```python
from build123d import *

# Parameters (mm, degrees)
F0_R     = 136.525
F0_R_2   = 2.15265
F0_R_3   = 127
F1_DEPTH = 3.175
F2_R     = 128.5875
F2_R_2   = 127
F3_DEPTH = 47.625
F5_DEPTH = 1.5875
F6_R     = 1.5
F6_R_2   = 6.35
F7_DEPTH = 1.5875


with BuildPart() as f1:
    # F0 (on Top) → F1 (new body)
    with BuildSketch(Plane.XY):
        Circle(F0_R)
        with Locations((-93.7314232637, -93.7314232637)):
            Circle(F0_R_2, mode=Mode.SUBTRACT)
        with Locations((93.7314232637, -93.7314232637)):
            Circle(F0_R_2, mode=Mode.SUBTRACT)
        with Locations((-93.7314232637, 93.7314232637)):
            Circle(F0_R_2, mode=Mode.SUBTRACT)
        Circle(F0_R_3, mode=Mode.SUBTRACT)
        with Locations((93.7314232637, 93.7314232637)):
            Circle(F0_R_2, mode=Mode.SUBTRACT)
    extrude(amount=F1_DEPTH)

    # F2 (on face) → F3 (join)
    with BuildSketch(Plane.XY.offset(3.175)):
        Circle(F2_R)
        Circle(F2_R_2, mode=Mode.SUBTRACT)
    extrude(amount=F3_DEPTH)

    # F4 (on face) → F5 (join)
    with BuildSketch(Plane.XY.offset(50.8)):
        with BuildLine():
            Line((-37.8011718568, 4.7625), (-126.9106717095, 4.7625))
            ThreePointArc((-126.9106717095, 4.7625), (-127, 0), (-126.9106717095, -4.7625))
            Line((-126.9106717095, -4.7625), (-37.8011718568, -4.7625))
            Line((-37.8011718568, -4.7625), (-37.8011718568, 4.7625))
        make_face()
        with BuildLine():
            ThreePointArc((127, 0), (126.9776659636, 2.3816688368), (126.9106717095, 4.7625))
            Line((126.9106717095, 4.7625), (37.8011718568, 4.7625))
            Line((37.8011718568, 4.7625), (37.8011718568, -4.7625))
            Line((37.8011718568, -4.7625), (126.9106717095, -4.7625))
            ThreePointArc((126.9106717095, -4.7625), (126.9776659636, -2.3816688368), (127, 0))
        make_face()
        with BuildLine():
            Line((-4.7625, -37.8011718568), (-4.7625, -126.9106717095))
            ThreePointArc((-4.7625, -126.9106717095), (0, -127), (4.7625, -126.9106717095))
            Line((4.7625, -126.9106717095), (4.7625, -37.8011718568))
            Line((4.7625, -37.8011718568), (-4.7625, -37.8011718568))
        make_face()
        with BuildLine():
            ThreePointArc((4.7625, 126.9106717095), (0, 127), (-4.7625, 126.9106717095))
            Line((-4.7625, 126.9106717095), (-4.7625, 37.8011718568))
            Line((-4.7625, 37.8011718568), (4.7625, 37.8011718568))
            Line((4.7625, 37.8011718568), (4.7625, 126.9106717095))
        make_face()
        with BuildLine():
            ThreePointArc((-4.7625, 37.8011718568), (-26.9407683632, 26.9407683632), (-37.8011718568, 4.7625))
            Line((-37.8011718568, 4.7625), (-37.8011718568, -4.7625))
            ThreePointArc((-37.8011718568, -4.7625), (-26.9407683632, -26.9407683632), (-4.7625, -37.8011718568))
            Line((-4.7625, -37.8011718568), (4.7625, -37.8011718568))
            ThreePointArc((4.7625, -37.8011718568), (26.9407683632, -26.9407683632), (37.8011718568, -4.7625))
            Line((37.8011718568, -4.7625), (37.8011718568, 4.7625))
            ThreePointArc((37.8011718568, 4.7625), (26.9407683632, 26.9407683632), (4.7625, 37.8011718568))
            Line((4.7625, 37.8011718568), (-4.7625, 37.8011718568))
        make_face()
    extrude(amount=-F5_DEPTH)

    # F6 (on face) → F7 (cut, through all)
    with BuildSketch(Plane.XY.offset(50.8)):
        with Locations((24.6957043329, 24.6957043329)):
            Circle(F6_R)
        with Locations((24.6957043329, -24.6957043329)):
            Circle(F6_R)
        with Locations((-24.6957043329, -24.6957043329)):
            Circle(F6_R)
        with Locations((-24.6957043329, 24.6957043329)):
            Circle(F6_R)
        Circle(F6_R_2)
    extrude(amount=-F7_DEPTH, mode=Mode.SUBTRACT)


solid = f1.part
```
Design review of the part built by this model. Coordinates are the model's own, in mm. A direction names the side the tool comes from. Round coordinates to 2 decimals unless told otherwise and drop trailing zeros. Write each loop counter-clockwise with the first axis right and the second up, starting at its lowest first coordinate (ties: lowest second). Pieces come first, ordered by that corner, then holes. Notation, with made-up numbers: (20, 58.25) -> (51, 58.25) arc R22 cw to (51, 93.25) -> close; hole circle Ø10 at (80, 88). An arc over 180 degrees is marked (long way). Write item = value, one per line. Start each with the question number.
1) Tool access review of faces 4 (the face through (27.19, 26.69, 50.02)), 5 (the face through (90.4, 91.7, 3.175)), 6 (the face through (121, -40, 0)), 7 (the face through (9, 1, 49.212)): name each direction out of +Z, -Z, +X, -X, +Y, -Y from which nothing blocks a thin tool from reaching the whole face with its end or side.
2) Take a section at C-C, the plane z = 35. State the section outline as (x, y) points (1 decimal).
3) Mouldability with a two-part tool opening along X and no side actions: class faces 1 (the face through (-10, 1, 50.8)), 2 (the face through (-102.043, -78.243, 26.654)), 3 (the face through (-26.69, 27.19, 50.02)) as +X half, -X half, draft (parallel to the pull), parting line (faces both ways), or undercut.
4) Clearance check with flat-ended pins moving along their axes: pin 1 (1.7 mm diameter, centred on x = -99, z = 50, fed in from -Y); pin 2 (10 mm diameter, centred on x = 70, z = 11, fed in from -Y); pin 3 (3.5 mm diameter, centred on x = 24.7, y = -24.7, fed in from -Z); pin 4 (2.5 mm diameter, centred on x = -24.7, y = 24.7, fed in from -Z). State where each tip first meets the part, or that it passes through.
5) Take a section at D-D, the plane x = -79.5. State the section outline as (y, z) points (1 decimal).
6) Wall thickness on probe 1 along X at (y, z) = (3, 7); probe 2 along X at (y, z) = (-112, 12.5); probe 3 along Y at (x, z) = (78.5, 39): over which ranges is each line inside the solid? List them lowest first. Write a range as from..to.
Results list:
q1.face_4 = +Z, -Z
q1.face_5 = +Z
q1.face_6 = -Z, +X, -X, +Y, -Y
q1.face_7 = -Z
q2.outline = circle Ø257.2 at (0, 0); hole circle Ø254 at (0, 0)
q3.face_1 = draft
q3.face_2 = parting line
q3.face_3 = undercut
q4.pin_1 = -83.07
q4.pin_2 = -110.95
q4.pin_3 = 49.21
q4.pin_4 = through
q5.outline = (-111, 0) -> (-99, 0) -> (-99, 50.8) -> (-101.1, 50.8) -> (-101.1, 3.2) -> (-111, 3.2) -> close; (-4.8, 49.2) -> (4.8, 49.2) -> (4.8, 50.8) -> (-4.8, 50.8) -> close; (99, 0) -> (111, 0) -> (111, 3.2) -> (101.1, 3.2) -> (101.1, 50.8) -> (99, 50.8) -> close
q6.probe_1 = -128.55..-126.96, 126.96..128.55
q6.probe_2 = -63.17..-59.87, 59.87..63.17
q6.probe_3 = -101.85..-99.83, 99.83..101.85
